Input: dimensioned drawing with shaded views. Units: mm. Origin: part minimum x, y, z. A direction names the side the tool comes from. Coordinates: 2 decimals unless noted, no trailing zeros. Order: outer loops, then holes, each group sorted by start corner. A loop starts at its lowest first (then second) coordinate and runs counter-clockwise, first axis right, second up. Notation, with made-up numbers: (65, -38) -> (120, -38) arc R28 cw to (120, -2) -> close; hole circle Ø10 at (41, 75). An arc over 180 degrees is marked (long way). Write item = value, one per line. Start each with the question number.
Item 1: Section query A-A (z = 15.5). Output: boundary loops of the cut face in (x, y).
Item 2: Section query C-C (y = 4.6). Output: boundary loops of the cut face in (x, z).
Item 3: Section query D-D (z = 1.5). Output: boundary loops of the cut face in (x, y), then the cut area to 3 significant figures.
Item 4: Ray query, line 1 along X through (y, z) = (4.4, 19); line 2 along Y through (x, z) = (27.5, 7.75); line 3 along Z through (x, y) = (28, 2.4). Return the intervals inside material, ascending. Write a range as [from, to].
Item 5: Contact query for flat-ended pins moving along their axis: pin 1 (0.5 mm diameter, centred on x = 30.5, y = 2.5, fed in from -Z); pin 2 (6.5 mm diameter, centred on x = 30, z = 10, fed in from +Y); pin 3 (2.5 mm diameter, centred on x = 30, z = 7.5, fed in from -Y). Output: stop coordinate, or through.
Item 6: Set-up query: the marked faces 1, 2 and 3. Return all of +Z, -Z, +X, -X, +Y, -Y with unobstructed straight access to the full face (end or side cutting, diameter ignored); none if empty.
Item 7: Section query B-B (x = 29.5). Output: boundary loops of the cut face in (y, z), then the cut area to 3 significant figures.
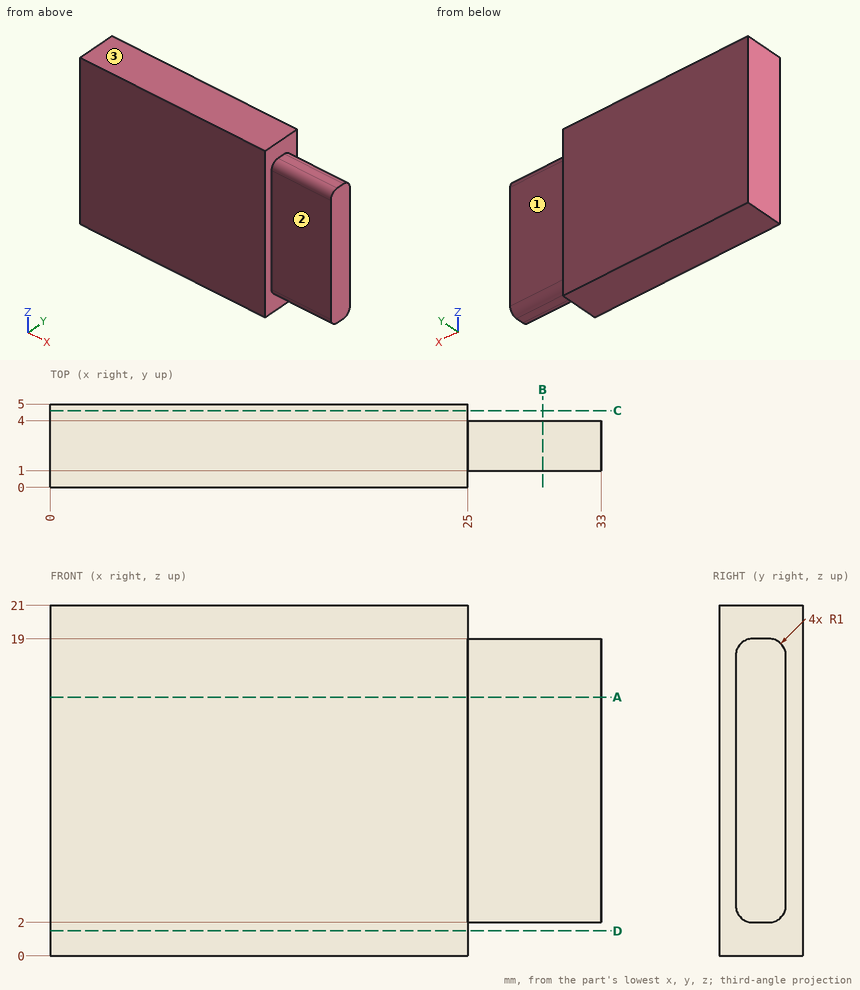
Computed:
q1.outline = (0, 0) -> (25, 0) -> (25, 1) -> (33, 1) -> (33, 4) -> (25, 4) -> (25, 5) -> (0, 5) -> close
q2.outline = (0, 0) -> (25, 0) -> (25, 21) -> (0, 21) -> close
q3.outline = (0, 0) -> (25, 0) -> (25, 5) -> (0, 5) -> close
q3.area = 125 mm^2
q4.line_1 = [0, 25]
q4.line_2 = [1, 4]
q4.line_3 = [2, 19]
q5.pin_1 = 2
q5.pin_2 = 4
q5.pin_3 = 1
q6.face_1 = +Z, -Z, +X, +Y
q6.face_2 = +Z, -Z, +X, -Y
q6.face_3 = +Z, +X, -X, +Y, -Y
q7.outline = (1, 3) arc R1 ccw to (2, 2) -> (3, 2) arc R1 ccw to (4, 3) -> (4, 18) arc R1 ccw to (3, 19) -> (2, 19) arc R1 ccw to (1, 18) -> close
q7.area = 50.1 mm^2
